Verification items for the finished model (mm, model axes). Face numbers are marked on the shaded views. A direction names the side the tool comes from. Coordinates: 2 decimals unless noted, no trailing zeros. Order: outer loops, then holes, each group sorted by start corner. A loop starts at its lowest first (then second) coordinate and runs counter-clockwise, first axis right, second up. Notation, with made-up numbers: (31, 19) - (39, 19) arc R19 ccw to (39, 46) - close; hole circle Ø2 at (43, 32.5). An arc over 180 degrees is marked (long way). Answer as CSV lines item,"result". Start each with the question number.
1. Set-up check for the marked faces 1 and 2: record each of +Z, -Z, +X, -X, +Y, -Y from which the full face is reachable in a straight line by a thin tool's end or side.
2. Material ranges on L1, parallel to X at y = 4.5, z = 1.75; L2, parallel to X at y = -3.25, z = 2; L3, parallel to Z at x = 9, y = 0, recorded low to high. Write a range as [from, to].
3. Section check A-A (x = 2.75). Record the cut outline in (y, z).
4. Go/stop test with flat-tipped pins: pin 1 (2 mm diameter, centred on y = -1.5, z = 4, fed in from +X); pin 2 (5 mm diameter, centred on y = 0, z = 2.5, fed in from -X); pin 3 (6 mm diameter, centred on x = 6.5, y = -2.5, fed in from +Z). Record where each tip stops, or that it passes through.
Autodesk Inventor part; units mm, degrees
ref_plane "YZ Plane" through (0, 0, 0) normal (1, 0, 0) x (0, 1, 0)
ref_plane "XZ Plane" through (0, 0, 0) normal (0, 1, 0) x (-1, 0, 0)
ref_plane "XY Plane" through (0, 0, 0) normal (0, 0, 1) x (1, 0, 0)
sketch "Sketch1" plane through (0, 0, 0) normal (0, 0, 1) x (1, 0, 0)
  line L0 (-8, 0) -> (20, 0)
  line L1 (16, 0) -> (16, 2.385)
  line L2 (16, 2.385) -> (15.385, 3)
  line L3 (15.385, 3) -> (0, 3)
  line L4 (0, 3) -> (0, 4.45)
  line L5 (0, 4.45) -> (-0.5, 4.45)
  line L6 (-0.5, 4.45) -> (-0.5, 5)
  line L7 (-0.5, 5) -> (-4, 5)
  line L8 (-4, 5) -> (-4, 0)
  point P0 (0, 0)
  dimension "d0" = 6
  dimension "d1" = 16
  dimension "d2" = 10
  dimension "d3" = 8.9
  dimension "d4" = 4
  dimension "d5" = 45
  dimension "d6" = 4.77
  dimension "d7" = 0.5
revolve "Revolution1" add sketch "Sketch1" angle 360 about axis through (-10, 0, 0) along (1, 0, 0)
sketch "Sketch2" plane through (-4, 0, 0) normal (-1, 0, 0) x (0, 0, 1)
  circle A0 centre (0, 0) radius 5
  line L0 (2.8868, 5) -> (5.7735, 0)
  line L1 (5.7735, 0) -> (2.8868, -5)
  line L2 (2.8868, -5) -> (-2.8868, -5)
  line L3 (-2.8868, -5) -> (-5.7735, 0)
  line L4 (-5.7735, 0) -> (-2.8868, 5)
  line L5 (-2.8868, 5) -> (2.8868, 5)
  point P0 (0, 5)
extrude "Extrusion1" add sketch "Sketch2" against normal up to surface (3.5 mm away)
sketch "Sketch3" plane through (0, 0, 0) normal (0, 0, 1) x (1, 0, 0)
  line L0 (-4, 5.55) -> (-0.5, 5.55)
  line L1 (-0.5, 5.55) -> (-0.5, 6.66)
  line L2 (-0.5, 6.66) -> (-4, 6.66)
  line L3 (-4, 6.66) -> (-4, 5.55)
  line L4 (-4.8, 0) -> (0.8, 0)
  line L5 (-4, 5) -> (-3.0416, 6.66)
  line L6 (-4, 5.55) -> (-4, 5)
  point P0 (0, 0)
  point P1 (-0.5, 5)
  dimension "d11" = 11.1
  dimension "d12" = 1.11
  dimension "d13" = 30
revolve "Revolution2" cut sketch "Sketch3" angle 360 about axis through (-10, 0, 0) along (1, 0, 0) contours L3 L2 L5 L0 | L0 L5 L6
thread "Thread1"
sketch "Sketch4" plane through (-4, 0, 0) normal (-1, 0, 0) x (0, 0, 1)
  circle A0 centre (0, 0) radius 3.75 construction
  spline S0 degree 2 poles (-2.4547, -1.0741) (-2.3544, -1.2038) (-2.112, -1.282) (-1.9755, -1.2387) knots 0 0 0 1 2 2 2
  spline S1 degree 2 poles (-1.9755, -1.2387) (-1.7677, -1.1728) (-1.5794, -0.7835) (-1.6577, -0.5365) knots 0 0 0 1 2 2 2
  spline S2 degree 2 poles (-1.6577, -0.5365) (-1.7371, -0.2866) (-2.1226, -0.0747) (-2.3304, -0.1406) knots 0 0 0 1 2 2 2
  spline S3 degree 2 poles (-2.3304, -0.1406) (-2.4626, -0.1826) (-2.6145, -0.3843) (-2.623, -0.5438) knots 0 0 0 1 2 2 2
  spline S4 degree 2 poles (-2.623, -0.5438) (-2.736, -0.3845) (-3.0498, -0.2826) (-3.227, -0.3389) knots 0 0 0 1 2 2 2
  spline S5 degree 2 poles (-3.227, -0.3389) (-3.4711, -0.4163) (-3.6941, -0.8677) (-3.6047, -1.1496) knots 0 0 0 1 2 2 2
  spline S6 degree 2 poles (-3.6047, -1.1496) (-3.5152, -1.4315) (-3.0713, -1.6712) (-2.8214, -1.5919) knots 0 0 0 1 2 2 2
  spline S7 degree 2 poles (-2.8214, -1.5919) (-2.6354, -1.5329) (-2.444, -1.2642) (-2.4547, -1.0741) knots 0 0 0 1 2 2 2
  spline S8 degree 2 poles (-2.8994, -1.3512) (-2.9996, -1.383) (-3.217, -1.348) (-3.3792, -1.1948) (-3.4133, -1.0873) knots 0 0 0 1 2 3 3 3
  spline S9 degree 2 poles (-3.4133, -1.0873) (-3.4668, -0.9187) (-3.319, -0.6335) (-3.1534, -0.581) knots 0 0 0 1 2 2 2
  spline S10 degree 2 poles (-3.1534, -0.581) (-2.9834, -0.527) (-2.6915, -0.6807) (-2.638, -0.8492) knots 0 0 0 1 2 2 2
  spline S11 degree 2 poles (-2.638, -0.8492) (-2.5855, -1.0149) (-2.7352, -1.2991) (-2.8994, -1.3512) knots 0 0 0 1 2 2 2
  spline S12 degree 2 poles (-2.0433, -0.9947) (-2.1784, -1.0376) (-2.4047, -0.9191) (-2.4486, -0.7811) knots 0 0 0 1 2 2 2
  spline S13 degree 2 poles (-2.4486, -0.7811) (-2.4914, -0.646) (-2.3759, -0.4206) (-2.2524, -0.3814) knots 0 0 0 1 2 2 2
  spline S14 degree 2 poles (-2.2524, -0.3814) (-2.1245, -0.3408) (-1.8929, -0.4608) (-1.8509, -0.593) knots 0 0 0 1 2 2 2
  spline S15 degree 2 poles (-1.8509, -0.593) (-1.808, -0.7282) (-1.9242, -0.9569) (-2.0433, -0.9947) knots 0 0 0 1 2 2 2
  line L0 (-3.75, -0.1349) -> (-3.471, -0.1349)
  line L1 (-3.471, -0.1349) -> (-3.471, 0.1441)
  line L2 (-3.471, 0.1441) -> (-3.75, 0.1441)
  line L3 (-3.75, 0.1441) -> (-3.75, -0.1349)
  spline S16 degree 2 poles (-2.6249, 0.538) (-2.6177, 0.3742) (-2.4648, 0.1705) (-2.3282, 0.1272) knots 0 0 0 1 2 2 2
  spline S17 degree 2 poles (-2.3282, 0.1272) (-2.1205, 0.0612) (-1.7421, 0.2706) (-1.6637, 0.5176) knots 0 0 0 1 2 2 2
  spline S18 degree 2 poles (-1.6637, 0.5176) (-1.5844, 0.7675) (-1.7772, 1.163) (-1.985, 1.2289) knots 0 0 0 1 2 2 2
  spline S19 degree 2 poles (-1.985, 1.2289) (-2.1172, 1.2709) (-2.3576, 1.1936) (-2.4566, 1.0683) knots 0 0 0 1 2 2 2
  spline S20 degree 2 poles (-2.4566, 1.0683) (-2.457, 1.2636) (-2.6546, 1.5278) (-2.8319, 1.5841) knots 0 0 0 1 2 2 2
  spline S21 degree 2 poles (-2.8319, 1.5841) (-3.076, 1.6615) (-3.5184, 1.4213) (-3.6079, 1.1394) knots 0 0 0 1 2 2 2
  spline S22 degree 2 poles (-3.6079, 1.1394) (-3.6973, 0.8576) (-3.4729, 0.4057) (-3.223, 0.3264) knots 0 0 0 1 2 2 2
  spline S23 degree 2 poles (-3.223, 0.3264) (-3.037, 0.2674) (-2.7257, 0.3765) (-2.6249, 0.538) knots 0 0 0 1 2 2 2
  spline S24 degree 2 poles (-3.1479, 0.568) (-3.2482, 0.5999) (-3.4056, 0.7538) (-3.4498, 0.9725) (-3.4156, 1.08) knots 0 0 0 1 2 3 3 3
  spline S25 degree 2 poles (-3.4156, 1.08) (-3.3621, 1.2486) (-3.0769, 1.3963) (-2.9113, 1.3438) knots 0 0 0 1 2 2 2
  spline S26 degree 2 poles (-2.9113, 1.3438) (-2.7413, 1.2898) (-2.5915, 0.996) (-2.645, 0.8274) knots 0 0 0 1 2 2 2
  spline S27 degree 2 poles (-2.645, 0.8274) (-2.6975, 0.6618) (-2.9837, 0.5159) (-3.1479, 0.568) knots 0 0 0 1 2 2 2
  spline S28 degree 2 poles (-2.243, 0.3656) (-2.3781, 0.4085) (-2.4947, 0.6358) (-2.4509, 0.7738) knots 0 0 0 1 2 2 2
  spline S29 degree 2 poles (-2.4509, 0.7738) (-2.408, 0.909) (-2.1836, 1.0265) (-2.0601, 0.9873) knots 0 0 0 1 2 2 2
  spline S30 degree 2 poles (-2.0601, 0.9873) (-1.9322, 0.9467) (-1.8122, 0.7151) (-1.8542, 0.5829) knots 0 0 0 1 2 2 2
  spline S31 degree 2 poles (-1.8542, 0.5829) (-1.897, 0.4477) (-2.1238, 0.3278) (-2.243, 0.3656) knots 0 0 0 1 2 2 2
  dimension "d17" = 7.5
extrude "Extrusion2" add sketch "Sketch4" along normal blind 0.1
equation "\"d7\" = 0.125 * d4"
equation "\"d12\" = 0.1 * d11"
properties part number "Sechskantschraube ISO 4017-M6x15-8.8" material "Steel"
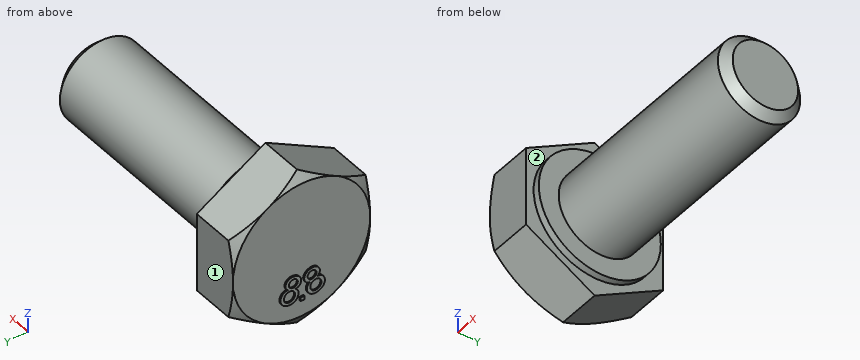
Evaluation:
1,face 1,"+Z, -Z, +X, -X, +Y"
1,face 2,"+X"
2,L1,"x = [-4, -0.5]"
2,L2,"x = [-4, 0]"
2,L3,"z = [-3, 3]"
3,outline,"circle Ø6 at (0, 0)"
4,pin 1,"stops at x = 0"
4,pin 2,"stops at x = -4"
4,pin 3,"stops at z = 3"
